from build123d import *

# Parameters (mm, degrees)
CYLINDER010_R      = 4.2
CYLINDER010_DEPTH  = 5
CYLINDER011_R      = 3.15
CYLINDER011_DEPTH  = 10
BOX016_W           = 22
BOX016_H           = 5
BOX016_DEPTH       = 14
CHAMFER006008_SIZE = 3
CHAMFER006012_SIZE = 0.4
BOX017_W           = 22
BOX017_H           = 5
BOX017_DEPTH       = 14
CHAMFER006013_SIZE = 3
CHAMFER006014_SIZE = 0.4
BOX018_W           = 7.8
BOX018_H           = 2
BOX018_DEPTH       = 14
BOX015_W           = 21.5
BOX015_H           = 5
BOX015_DEPTH       = 14
CHAMFER006009_SIZE = 3
CHAMFER006015_SIZE = 0.4


with BuildPart() as cylinder010:
    # Cylinder010 → Cylinder010 (new body)
    with BuildSketch(Plane(origin=(-14, -5, 7), x_dir=(1, 0, 0), z_dir=(0, 1, 0))):
        Circle(CYLINDER010_R)
    extrude(amount=CYLINDER010_DEPTH)


with BuildPart() as cylinder011:
    # Cylinder011 → Cylinder011 (new body)
    with BuildSketch(Plane(origin=(15, 8, 7), x_dir=(1, 0, 0), z_dir=(0, -1, 0))):
        Circle(CYLINDER011_R)
    extrude(amount=CYLINDER011_DEPTH)


with BuildPart() as chamfer006012:
    # Box016 → Box016 (new body)
    with BuildSketch(Plane(origin=(-22, 0, 0), x_dir=(1, 0, 0), z_dir=(0, 0, 1))):
        with Locations((11, 2.5)):
            Rectangle(BOX016_W, BOX016_H)
    extrude(amount=BOX016_DEPTH)

    # Chamfer006008
    chamfer006008_edges = [chamfer006012.edges().sort_by_distance(p)[0] for p in [
        (-22, 2.5, 14),
        (-22, 2.5, 0),
    ]]
    chamfer(chamfer006008_edges, length=CHAMFER006008_SIZE)

    # Chamfer006012
    chamfer006012_edges = [chamfer006012.edges().sort_by_distance(p)[0] for p in [
        (-22, 5, 7),
        (-20.5, 5, 1.5),
        (-20.5, 5, 12.5),
        (-9.5, 5, 0),
        (-9.5, 5, 14),
    ]]
    chamfer(chamfer006012_edges, length=CHAMFER006012_SIZE)


with BuildPart() as chamfer006014:
    # Box017 → Box017 (new body)
    with BuildSketch(Plane.XY):
        with Locations((11, 2.5)):
            Rectangle(BOX017_W, BOX017_H)
    extrude(amount=BOX017_DEPTH)

    # Chamfer006013
    chamfer006013_edges = [chamfer006014.edges().sort_by_distance(p)[0] for p in [
        (22, 2.5, 14),
        (22, 2.5, 0),
    ]]
    chamfer(chamfer006013_edges, length=CHAMFER006013_SIZE)

    # Chamfer006014
    chamfer006014_edges = [chamfer006014.edges().sort_by_distance(p)[0] for p in [
        (22, 5, 7),
        (20.5, 5, 1.5),
        (20.5, 5, 12.5),
        (9.5, 5, 0),
        (9.5, 5, 14),
    ]]
    chamfer(chamfer006014_edges, length=CHAMFER006014_SIZE)


with BuildPart() as cube017:
    # Box018 → Box018 (new body)
    with BuildSketch(Plane(origin=(11.1, -1, 0), x_dir=(1, 0, 0), z_dir=(0, 0, 1))):
        with Locations((3.9, 1)):
            Rectangle(BOX018_W, BOX018_H)
    extrude(amount=BOX018_DEPTH)


with BuildPart() as chamfer006015:
    # Box015 → Box015 (new body)
    with BuildSketch(Plane(origin=(-22, -5, 0), x_dir=(1, 0, 0), z_dir=(0, 0, 1))):
        with Locations((10.75, 2.5)):
            Rectangle(BOX015_W, BOX015_H)
    extrude(amount=BOX015_DEPTH)

    # Chamfer006009
    chamfer006009_edges = [chamfer006015.edges().sort_by_distance(p)[0] for p in [
        (-22, -2.5, 14),
        (-22, -2.5, 0),
    ]]
    chamfer(chamfer006009_edges, length=CHAMFER006009_SIZE)

    # Fusion005: union Chamfer006012, Chamfer006014, Cube017
    add(chamfer006012.part)
    add(chamfer006014.part)
    add(cube017.part)

    # Cut010011008009003016026008003008002: cut Cylinder011
    add(cylinder011.part, mode=Mode.SUBTRACT)

    # Cut010011008009003016026008003008003: cut Cylinder010
    add(cylinder010.part, mode=Mode.SUBTRACT)

    # Chamfer006015
    chamfer006015_edges = [chamfer006015.edges().sort_by_distance(p)[0] for p in [
        (-18.2, -5, 7),
    ]]
    chamfer(chamfer006015_edges, length=CHAMFER006015_SIZE)


solid = chamfer006015.part
Geometry check sheet. Reference: the model listing, model coordinates, mm. A direction names the side the tool comes from. Round coordinates to 2 decimals unless told otherwise and drop trailing zeros. Loops run counter-clockwise (first coordinate to the right, second up) from the corner with the lowest first, then second, coordinate; pieces in that order, holes last. Notation, with made-up numbers: (-36.5, 69.5) -> (-11.5, 69.5) arc R7 ccw to (-11.5, 76.5) -> close; hole circle Ø9 at (1, -12.75). An arc over 180 degrees is marked (long way). Answer as a JSON object with one key per item and string values. Group by question number.
Item 1: Release check for a two-part mould opening along Z. For faces 4 (the face through (-9, -5, 7)), 5 (the face through (-14.91, -2.33, 11.1)), 6 (the face through (-20, 0, 1)) record: pulls with the +Z half, pulls with the -Z half, needs draft (parallel to the pull), parting line crosses it, or undercut.
Item 2: Depth check by flat-ended pin: pin 1 Ø4 at (x, z) = (-16, 8.5) entering from -Y; pin 2 Ø1.5 at (y, z) = (-1.5, 6) entering from +X; pin 3 Ø4 at (x, z) = (14, 10) entering from -Y; pin 4 Ø5.5 at (x, z) = (15, 7) entering from -Y. Enter the tip coordinate at first touch or a pass-through.
Item 3: Cross-section at D-D, the plane y = -3.5. Record the cut outline in (x, z), plus the area to 3 significant figures.
Item 4: Cross-section at C-C, the plane z = 7. Record the cut outline in (x, y).
Item 5: Set-up check for faces 1 (the face through (5, 0, 7)), 2 (the face through (20, 2, 13)), 3 (the face through (14.1, -1, 3.8)): record each of +Z, -Z, +X, -X, +Y, -Y from which the full face is reachable in a straight line by a thin tool's end or side.
Item 6: Thickness scan on line 1 along X through (y, z) = (1.05, 7); line 2 along X through (y, z) = (-2.95, 7); line 3 along Z through (x, y) = (15, 1.25). Record the ranges inside material, lowest first.
Item 7: Cross-section at B-B, the plane x = 15. Record the cut outline in (y, z).
Item 8: Cross-section at A-A, the plane y = -0.5. Record the cut outline in (x, z).
Determined:
{
 "1": {"face 4": "needs draft", "face 5": "undercut", "face 6": "pulls with the -Z half"},
 "2": {"pin 1": "stops at y = -4.9", "pin 2": "stops at x = 18.9", "pin 3": "stops at y = -1", "pin 4": "passes through"},
 "3": {"outline": "(-22, 3) -> (-19, 0) -> (-0.5, 0) -> (-0.5, 14) -> (-19, 14) -> (-22, 11) -> close; hole circle Ø8.4 at (-14, 7)", "area": "237 mm²"},
 "4": {"outline": "(-22, -5) -> (-18.6, -5) -> (-18.2, -4.6) -> (-18.2, 0) -> (-9.8, 0) -> (-9.8, -4.6) -> (-9.4, -5) -> (-0.5, -5) -> (-0.5, 0) -> (11.1, 0) -> (11.1, -1) -> (11.85, -1) -> (11.85, 5) -> (-21.6, 5) -> (-22, 4.6) -> close; (18.15, -1) -> (18.9, -1) -> (18.9, 0) -> (22, 0) -> (22, 4.6) -> (21.6, 5) -> (18.15, 5) -> close"},
 "5": {"face 1": "+Z, -Z, -Y", "face 2": "+Z, +X, +Y, -Y", "face 3": "+Z, -Z, +X, -Y"},
 "6": {"line 1": "x = -22 to 11.85, 18.15 to 22", "line 2": "x = -22 to -18.2, -9.8 to -0.5", "line 3": "z = 0 to 3.85, 10.15 to 14"},
 "7": {"outline": "(-1, 0) -> (4.6, 0) -> (5, 0.4) -> (5, 3.85) -> (-1, 3.85) -> close; (-1, 10.15) -> (5, 10.15) -> (5, 13.6) -> (4.6, 14) -> (-1, 14) -> close"},
 "8": {"outline": "(-22, 3) -> (-19, 0) -> (-0.5, 0) -> (-0.5, 14) -> (-19, 14) -> (-22, 11) -> close; (11.1, 0) -> (18.9, 0) -> (18.9, 14) -> (11.1, 14) -> close; hole circle Ø8.4 at (-14, 7); hole circle Ø6.3 at (15, 7)"}
}
